Answer from the drawing. Dimensions are ordinates in mm from the lowest x, y and z of the part. A direction names the side the tool comes from. Coordinates: 2 decimals unless noted, no trailing zeros. Write each loop counter-clockwise with the first axis right and the second up, starting at its lowest first coordinate (ties: lowest second). Pieces come first, ordered by that corner, then holes.
(1) Section D-D on y = 24 is taken. Write down the section's boundary in (x, z), then the cut area to 3 significant figures.
(2) Which of the six approach directions +Z, -Z, +X, -X, +Y, -Y give full straight-line access (tool end or side, diameter ignored) to the marked faces 4 and 5?
(3) Section B-B on x = 21 is taken. Write down the section's boundary in (y, z), then the cut area to 3 significant figures.
(4) Section A-A on y = 11 is taken. Write down the section's boundary in (x, z), then the cut area to 3 significant figures.
(5) Section C-C on z = 6.5 is taken. Write down the section's boundary in (x, y).
(6) The mould has two halves that part along Z. Classify the marked faces 1, 2 and 3: +Z half, -Z half, draft (parallel to the pull), parting line (faces both ways), or undercut.
(7) Given pin 1 (0.6 mm diameter, centred on x = 16.5, z = 1, fed in from +Y); pin 2 (6 mm diameter, centred on x = 24.5, z = 7, fed in from -Y); pin 3 (1.6 mm diameter, centred on x = 30.5, z = 15, fed in from -Y), each flat-ended and moving along its own axis, determine where each tip first touches the part or whether it passes through.
(8) Find the intervals of material crossed by probe 1 along Z at (x, y) = (2.5, 16), in increasing order.
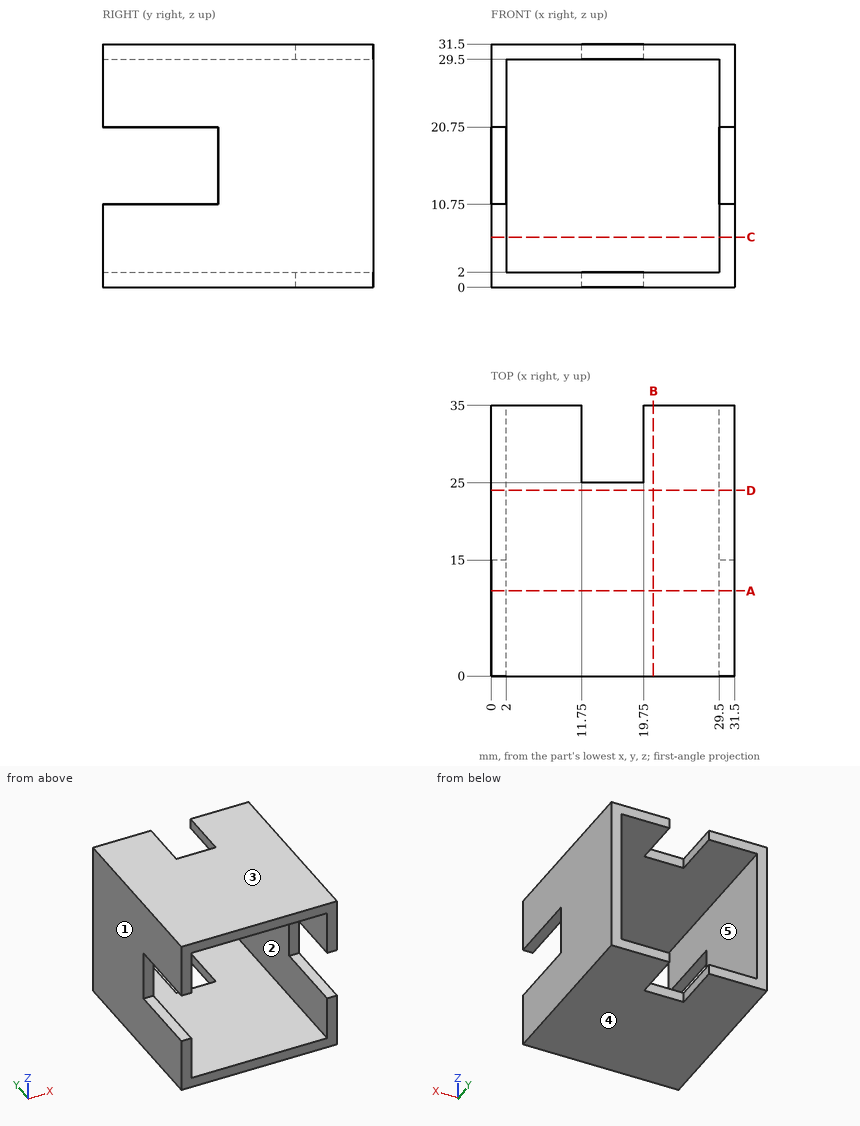
Response:
1. outline: (0, 0) - (31.5, 0) - (31.5, 31.5) - (0, 31.5) - close; hole (2, 2) - (29.5, 2) - (29.5, 29.5) - (2, 29.5) - close
1. area: 236 mm2
2. face 4: -Z, +X, -X, +Y, -Y
2. face 5: +Y, -Y
3. outline: (0, 0) - (35, 0) - (35, 2) - (0, 2) - close; (0, 29.5) - (35, 29.5) - (35, 31.5) - (0, 31.5) - close
3. area: 140 mm2
4. outline: (0, 0) - (31.5, 0) - (31.5, 10.75) - (29.5, 10.75) - (29.5, 2) - (2, 2) - (2, 10.75) - (0, 10.75) - close; (0, 20.75) - (2, 20.75) - (2, 29.5) - (29.5, 29.5) - (29.5, 20.75) - (31.5, 20.75) - (31.5, 31.5) - (0, 31.5) - close
4. area: 196 mm2
5. outline: (0, 0) - (2, 0) - (2, 35) - (0, 35) - close; (29.5, 0) - (31.5, 0) - (31.5, 35) - (29.5, 35) - close
6. face 1: draft
6. face 2: undercut
6. face 3: +Z half
7. pin 1: stops at y = 25
7. pin 2: passes through
7. pin 3: stops at y = 15
8. probe 1: z = 0 to 2, 29.5 to 31.5
